Here's the drawing with two shaded views (mm, measured from the low corner). I have some questions. Coordinates: 2 decimals unless noted, no trailing zeros. Write each loop counter-clockwise with the first axis right and the second up, starting at its lowest first coordinate (ties: lowest second). Pieces come first, ordered by that corner, then holes.
Item 1: If I drill on line 1 (Y direction, x = 21.75, z = 75); line 2 (Z direction, x = 8.5, y = 450); line 3 (Z direction, x = 18, y = 37), over which ranges is the centre line in solid material (lowest first)?
Item 2: If we section it at D-D (y = 263): Please give me the cut outline in (x, z), then the cut area to 3 significant figures.
Item 3: If we section it at B-B (y = 449.33): Please give me the cut outline in (x, z).
Item 4: If we section it at A-A (z = 75): Please give me the cut outline in (x, y), then the cut area to 3 significant figures.
Item 5: We'd pull the mould along Z, two halves only. Please class the marked faces 1, 2 and 3: +Z half, -Z half, draft (parallel to the pull), parting line (faces both ways), or undercut.
Item 6: I'm going to push flat-ended pins straight in: pin 1 Ø4 at (y, z) = (79.5, 63.5) entering from +X; pin 2 Ø24 at (y, z) = (37.5, 75) entering from -X; pin 3 Ø1.5 at (y, z) = (337, 51) entering from -X. Where does each tip first touch, or does it pass through?
Item 7: If we section it at C-C (x = 31.5): Please give me the cut outline in (y, z), then the cut area to 3 significant figures.
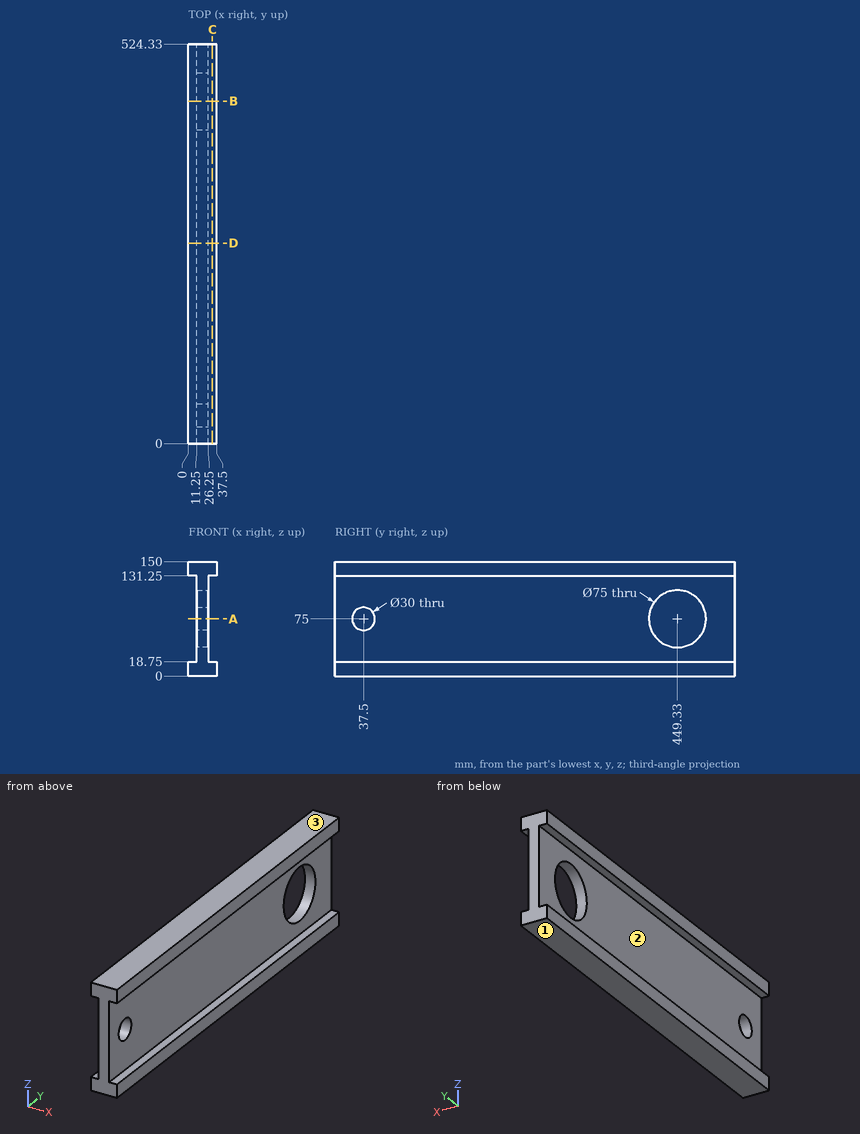
Answer list:
1. line 1: y = 0 to 22.5, 52.5 to 411.83, 486.83 to 524.33
1. line 2: z = 0 to 18.75, 131.25 to 150
1. line 3: z = 0 to 60.01, 89.99 to 150
2. outline: (0, 0) - (37.5, 0) - (37.5, 18.75) - (26.25, 18.75) - (26.25, 131.25) - (37.5, 131.25) - (37.5, 150) - (0, 150) - (0, 131.25) - (11.25, 131.25) - (11.25, 18.75) - (0, 18.75) - close
2. area: 3,090 mm2
3. outline: (0, 0) - (37.5, 0) - (37.5, 18.75) - (26.25, 18.75) - (26.25, 37.5) - (11.25, 37.5) - (11.25, 18.75) - (0, 18.75) - close; (0, 131.25) - (11.25, 131.25) - (11.25, 112.5) - (26.25, 112.5) - (26.25, 131.25) - (37.5, 131.25) - (37.5, 150) - (0, 150) - close
4. outline: (11.25, 0) - (26.25, 0) - (26.25, 22.5) - (11.25, 22.5) - close; (11.25, 52.5) - (26.25, 52.5) - (26.25, 411.83) - (11.25, 411.83) - close; (11.25, 486.83) - (26.25, 486.83) - (26.25, 524.33) - (11.25, 524.33) - close
4. area: 6,290 mm2
5. face 1: -Z half
5. face 2: undercut
5. face 3: +Z half
6. pin 1: stops at x = 26.25
6. pin 2: passes through
6. pin 3: stops at x = 11.25
7. outline: (0, 0) - (524.33, 0) - (524.33, 18.75) - (0, 18.75) - close; (0, 131.25) - (524.33, 131.25) - (524.33, 150) - (0, 150) - close
7. area: 19,700 mm2
